Source: CAD feature listing. Evaluate the final solid. Frame: model axes, mm. Face numbers are marked on the shaded views. A direction names the side the tool comes from. Coordinates: 2 decimals unless noted, no trailing zeros. Loops run counter-clockwise (first coordinate to the right, second up) from the corner with the lowest first, then second, coordinate; pieces in that order, holes last.
Item 1: Pull-direction query (Y, two-part tool) for the marked faces 1, 2 and 3; classes: +Y half, -Y half, draft (parallel to the pull), parting line (faces both ways), or undercut.
Item 2: Line query: probe 1 along Y at (x, z) = (9, -5); probe 2 along Y at (x, z) = (13.5, 3.25); probe 3 along Z at (x, y) = (6.75, 16). Output: solid intervals per line, ascending.
Item 3: Section query C-C, the plane y = 17.5. Return the cut outline in (x, z), then the cut area to 3 significant figures.
Item 4: Reachability of the marked faces 4, 5, 6, 7 and 8 from +Z, -Z, +X, -X, +Y, -Y: full face, straight path, thin tool, end or side. Return the list, or none.
Item 5: Pin query (flat end, axial travel): pin 1 Ø10 at (x, y) = (12, 29) entering from -Z; pin 2 Ø1.5 at (y, z) = (15, -1) entering from -X; pin 3 Ø6 at (x, y) = (14, 11.5) entering from +Z. Return the tip coordinate at first contact, or that it passes through.
Item 6: Section query B-B, the plane x = 7. Return the cut outline in (y, z), then the cut area to 3 significant figures.
Item 7: Section query A-A, the plane z = 0. Return the cut outline in (x, y), then the cut area to 3 significant figures.
```python
from build123d import *

# Parameters (mm, degrees)
CHAMFER1_SIZE = 1.5


with BuildPart() as part:
    # Sketch1 → Revolve1 (revolve)
    with BuildSketch(Plane.XY):
        Polygon((7, 0), (0, 0), (0, 6), (-2, 6), (-2, 9), (0, 9), (0, 30), (3.25, 30), (3.25, 34), (0, 34), (0, 43), (7, 43), align=None)
    revolve(axis=Axis((7, 43, 0), (0, -1, 0)))

    # Chamfer1
    chamfer1_edges = [part.edges().sort_by_distance(p)[0] for p in [
        (14, 43, 0),
    ]]
    chamfer(chamfer1_edges, length=CHAMFER1_SIZE)


solid = part.part
```
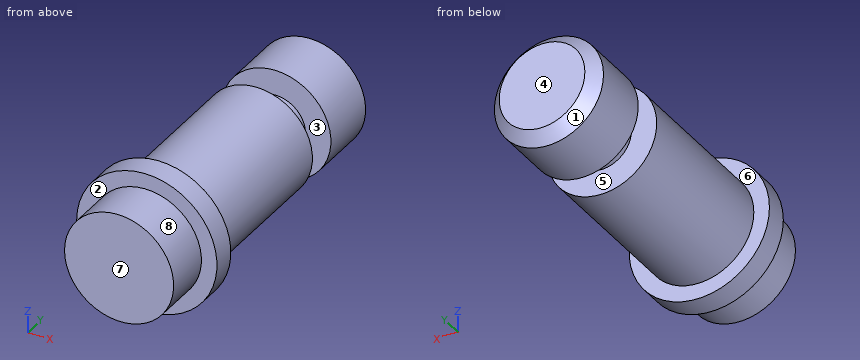
Verdict:
1. face 1: +Y half
1. face 2: -Y half
1. face 3: undercut
2. probe 1: y = 0 to 30, 34 to 43
2. probe 2: y = 6 to 9
2. probe 3: z = -7 to 7
3. outline: circle Ø14 at (7, 0)
3. area: 154 mm2
4. face 4: +Z, -Z, +X, -X, +Y
4. face 5: none
4. face 6: +Y
4. face 7: +Z, -Z, +X, -X, -Y
4. face 8: -Y
5. pin 1: stops at z = -7
5. pin 2: stops at x = 0
5. pin 3: stops at z = 7.24
6. outline: (0, -7) - (6, -7) - (6, -9) - (9, -9) - (9, -7) - (30, -7) - (30, -3.75) - (34, -3.75) - (34, -7) - (41.5, -7) - (43, -5.5) - (43, 5.5) - (41.5, 7) - (34, 7) - (34, 3.75) - (30, 3.75) - (30, 7) - (9, 7) - (9, 9) - (6, 9) - (6, 7) - (0, 7) - close
6. area: 586 mm2
7. outline: (-2, 6) - (0, 6) - (0, 0) - (14, 0) - (14, 6) - (16, 6) - (16, 9) - (14, 9) - (14, 30) - (10.75, 30) - (10.75, 34) - (14, 34) - (14, 41.5) - (12.5, 43) - (1.5, 43) - (0, 41.5) - (0, 34) - (3.25, 34) - (3.25, 30) - (0, 30) - (0, 9) - (-2, 9) - close
7. area: 586 mm2
